Could you check a few things on this model? Use its own coordinates, in mm. Face numbers are marked on the shaded views. A direction names the side the tool comes from. Give positions to 0.01 mm unless a question says otherwise; leave off trailing zeros. Write each loop counter-clockwise with the first axis right and the second up, starting at its lowest first coordinate (ties: lowest second). Pieces come first, ordered by that corner, then holes. Notation, with made-up numbers: (54.25, 78) -> (107.25, 78) arc R25 cw to (107.25, 94) -> close; hole circle Ø6 at (-6, 27.5). An arc over 180 degrees is marked (long way). One line per question, with ' | ' between items.
from build123d import *

# Parameters (mm, degrees)
SKETCH1_W                = 90.006
SKETCH1_H                = 90
SKETCH1_R                = 16.2
ALPHASENSE_HOUSING_DEPTH = 5
SKETCH2_W                = 90.006
SKETCH2_H                = 90
SKETCH2_R                = 9.5
CHAMBER_HOUSING_DEPTH    = 13
SKETCH3_W                = 90.006
SKETCH3_H                = 90
BASE_DEPTH               = 6
SKETCH5_R                = 5.9
DRILL_DEPTH              = 10
SKETCH6_R                = 5.9
DRILL2_DEPTH             = 10
SKETCH7_R                = 5.9
DRILL3_DEPTH             = 10
SKETCH8_R                = 5.9
INLETDRILL_DEPTH         = 10
SKETCH10_R               = 5.9
DRILL5_DEPTH             = 10
SKETCH11_R               = 5.9
OUTLEDRILL_DEPTH         = 10
SKETCH12_R               = 1.75
CLIPPINGTHREADS_DEPTH    = 10
SKETCH13_R               = 4
CUT_EXTRUDE1_DEPTH       = 35.003
SKETCH14_R               = 4
CUT_EXTRUDE2_DEPTH       = 16.098
SKETCH15_R               = 4
CUT_EXTRUDE3_DEPTH       = 22.255579
SKETCH16_R               = 4
CUT_EXTRUDE4_DEPTH       = 22.255579
SKETCH17_R               = 4
CUT_EXTRUDE5_DEPTH       = 16.098
SKETCH18_R               = 4
CUT_EXTRUDE6_DEPTH       = 15


with BuildPart() as part:
    # Sketch1 → Alphasense_housing (new body)
    with BuildSketch(Plane(origin=(0, 0, 0), x_dir=(1, 0, 0), z_dir=(0, 1, 0))):
        with Locations((0, 1.829613678)):
            Rectangle(SKETCH1_W, SKETCH1_H)
        with Locations((0, 21.829613678)):
            Circle(SKETCH1_R, mode=Mode.SUBTRACT)
        with Locations((-18.905, -10.914806839)):
            Circle(SKETCH1_R, mode=Mode.SUBTRACT)
        with Locations((18.905, -10.914806839)):
            Circle(SKETCH1_R, mode=Mode.SUBTRACT)
    extrude(amount=ALPHASENSE_HOUSING_DEPTH)

    # Sketch2 → Chamber_housing (add)
    with BuildSketch(Plane.XZ):
        with Locations((0, -1.829613678)):
            Rectangle(SKETCH2_W, SKETCH2_H)
        with Locations((-18.905, 10.914806839)):
            Circle(SKETCH2_R, mode=Mode.SUBTRACT)
        with Locations((18.905, 10.914806839)):
            Circle(SKETCH2_R, mode=Mode.SUBTRACT)
        with Locations((0, -21.829613678)):
            Circle(SKETCH2_R, mode=Mode.SUBTRACT)
    extrude(amount=CHAMBER_HOUSING_DEPTH)

    # Sketch3 → Base (add)
    with BuildSketch(Plane.XZ.offset(13)):
        with Locations((0, -1.829613678)):
            Rectangle(SKETCH3_W, SKETCH3_H)
    extrude(amount=BASE_DEPTH)

    # Sketch5 → Drill (cut)
    with BuildSketch(Plane.ZY.offset(45.003)):
        with Locations((20.414806839, -10)):
            Circle(SKETCH5_R)
    extrude(amount=-DRILL_DEPTH, mode=Mode.SUBTRACT)

    # Sketch6 → Drill2 (cut)
    with BuildSketch(Plane.XY.offset(43.170386322)):
        with Locations((-9.405, -10)):
            Circle(SKETCH6_R)
    extrude(amount=-DRILL2_DEPTH, mode=Mode.SUBTRACT)

    # Sketch7 → Drill3 (cut)
    with BuildSketch(Plane.XY.offset(43.170386322)):
        with Locations((9.405, -10)):
            Circle(SKETCH7_R)
    extrude(amount=-DRILL3_DEPTH, mode=Mode.SUBTRACT)

    # Sketch8 → InletDrill (cut)
    with BuildSketch(Plane(origin=(45.003, 0, 0), x_dir=(0, 0, -1), z_dir=(1, 0, 0))):
        with Locations((-20.414806839, -10)):
            Circle(SKETCH8_R)
    extrude(amount=-INLETDRILL_DEPTH, mode=Mode.SUBTRACT)

    # Sketch10 → Drill5 (cut)
    with BuildSketch(Plane.ZY.offset(45.003)):
        with Locations((-12.329613678, -10)):
            Circle(SKETCH10_R)
    extrude(amount=-DRILL5_DEPTH, mode=Mode.SUBTRACT)

    # Sketch11 → OutleDrill (cut)
    with BuildSketch(Plane(origin=(0, 0, -46.829613678), x_dir=(-1, 0, 0), z_dir=(0, 0, -1))):
        with Locations((9.5, -10)):
            Circle(SKETCH11_R)
    extrude(amount=-OUTLEDRILL_DEPTH, mode=Mode.SUBTRACT)

    # Sketch12 → ClippingThreads (cut)
    with BuildSketch(Plane(origin=(0, 5, 0), x_dir=(1, 0, 0), z_dir=(0, 1, 0))):
        with Locations((-35, 36.829613678)):
            Circle(SKETCH12_R)
        with Locations((35, 36.829613678)):
            Circle(SKETCH12_R)
        with Locations((-35, -35.914806839)):
            Circle(SKETCH12_R)
        with Locations((35, -35.914806839)):
            Circle(SKETCH12_R)
    extrude(amount=-CLIPPINGTHREADS_DEPTH, mode=Mode.SUBTRACT)

    # Sketch13 → Cut-Extrude1 (cut)
    with BuildSketch(Plane.ZY.offset(35.003)):
        with Locations((-12.329613678, -10)):
            Circle(SKETCH13_R)
    extrude(amount=-CUT_EXTRUDE1_DEPTH, mode=Mode.SUBTRACT)

    # Sketch14 → Cut-Extrude2 (cut)
    with BuildSketch(Plane.ZY.offset(35.003)):
        with Locations((20.414806839, -10)):
            Circle(SKETCH14_R)
    extrude(amount=-CUT_EXTRUDE2_DEPTH, mode=Mode.SUBTRACT)

    # Sketch15 → Cut-Extrude3 (cut)
    with BuildSketch(Plane.XY.offset(33.170386322)):
        with Locations((-9.405, -10)):
            Circle(SKETCH15_R)
    extrude(amount=-CUT_EXTRUDE3_DEPTH, mode=Mode.SUBTRACT)

    # Sketch16 → Cut-Extrude4 (cut)
    with BuildSketch(Plane.XY.offset(33.170386322)):
        with Locations((9.405, -10)):
            Circle(SKETCH16_R)
    extrude(amount=-CUT_EXTRUDE4_DEPTH, mode=Mode.SUBTRACT)

    # Sketch17 → Cut-Extrude5 (cut)
    with BuildSketch(Plane(origin=(35.003, 0, 0), x_dir=(0, 0, -1), z_dir=(1, 0, 0))):
        with Locations((-20.414806839, -10)):
            Circle(SKETCH17_R)
    extrude(amount=-CUT_EXTRUDE5_DEPTH, mode=Mode.SUBTRACT)

    # Sketch18 → Cut-Extrude6 (cut)
    with BuildSketch(Plane(origin=(0, 0, -36.829613678), x_dir=(-1, 0, 0), z_dir=(0, 0, -1))):
        with Locations((9.5, -10)):
            Circle(SKETCH18_R)
    extrude(amount=-CUT_EXTRUDE6_DEPTH, mode=Mode.SUBTRACT)


solid = part.part
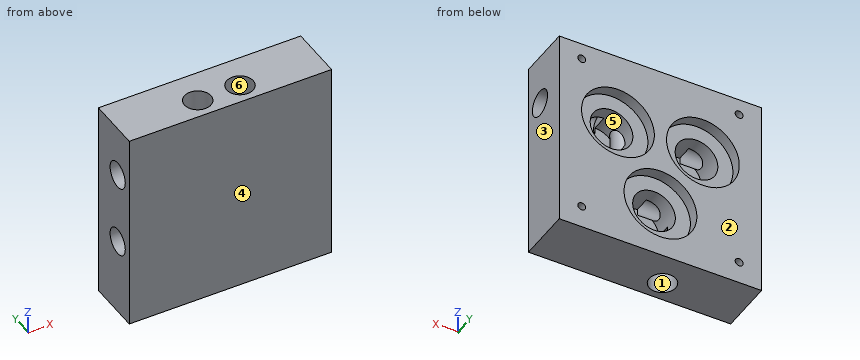
Q1. Imagine slicing it at D-D on y = -10. Count the separate pieces of the cut face and the enclosed holes in it, and give its area (3 significant figures).
Answer below:
separate pieces: 4 | enclosed holes: 0 | area: 5,660 mm^2
Q2. If I drill on line 1 along X through (y, z) = (-10.25, 23) (3 decimals); line 2 along Z through (x, y) = (-35, -1.75); line 3 along X through (y, z) = (-9.75, 28), over which ranges is the centre line in solid material (lowest first)?
Answer below:
line 1: x = -18.905 to -13.397, -5.413 to 5.413, 13.397 to 18.905 | line 2: z = -46.83 to -38.58, -35.08 to 34.16, 37.66 to 43.17 | line 3: x = -45 to -13.4, -5.41 to 5.41, 13.4 to 45
Q3. Imagine slicing it at A-A on x = 39.5. Please give me the cut outline in (y, z), and give its area (3 significant figures).
Answer below:
outline: (-19, -46.83) -> (5, -46.83) -> (5, 43.17) -> (-19, 43.17) -> close; hole circle Ø11.8 at (-10, 20.41) | area: 2,050 mm^2
Q4. On a 3-axis mill with a long thin cutter (end or side, diameter ignored), from which of +Z, -Z, +X, -X, +Y, -Y can I reach the whole of each face in a straight line? I mean the marked faces 4, 5 and 6. Say none if no direction works.
Answer below:
face 4: +Z, -Z, +X, -X, -Y | face 5: +Y | face 6: +Z
Q5. Imagine slicing it at B-B on z = 31. Please give me the cut outline in (x, y) (3 decimals), and give its area (3 significant figures).
Answer below:
outline: (-45.003, -19) -> (45.003, -19) -> (45.003, 5) -> (-45.003, 5) -> close; hole circle Ø8 at (-9.405, -10); hole circle Ø8 at (9.405, -10) | area: 2,060 mm^2
Q6. If we mould it in two halves opening along X, with no side actions, what happens to the marked faces 1, 2 and 3? For each: +X half, -X half, draft (parallel to the pull), parting line (faces both ways), or undercut.
Answer below:
face 1: undercut | face 2: draft | face 3: +X half
Q7. Will these pins go through, and if not, where does the flat tip stop? pin 1 (3.5 mm diameter, centred on x = 10, y = -11.5, fed in from +Z); pin 2 (9.5 mm diameter, centred on x = -14.5, z = 14, fed in from +Y); pin 3 (13 mm diameter, centred on y = -10, z = 20.41, fed in from +X); pin 4 (9 mm diameter, centred on y = -10, z = 20.41, fed in from +X).
Answer below:
pin 1: stops at z = 10.91 | pin 2: stops at y = 0 | pin 3: stops at x = 45 | pin 4: stops at x = 35
Q8. Imagine slicing it at C-C on x = 22. Please give me the cut outline in (y, z), and give its area (3 significant figures).
Answer below:
outline: (-19, -46.83) -> (5, -46.83) -> (5, -4.99) -> (0, -4.99) -> (0, 1.93) -> (-13, 1.93) -> (-13, 17.77) arc R4 cw (long way) to (-6.03, 19.9) -> (0, 19.9) -> (0, 26.82) -> (5, 26.82) -> (5, 43.17) -> (-19, 43.17) -> close | area: 1,740 mm^2
